Verification items for the finished model (mm, model axes). Face numbers are marked on the shaded views. Give positions to 0.01 mm unless a question says otherwise; leave off trailing zeros. Order: outer loops, then holes, each group sorted by start corner. A loop starts at its lowest first (then second) coordinate and runs counter-clockwise, first axis right, second up.
from build123d import *

# Parameters (mm, degrees)
F1_DEPTH = 100
F2_R     = 15
F3_DEPTH = 100.001
F4_R     = 15
F5_DEPTH = 100.001
F6_R     = 15
F7_DEPTH = 100.001


with BuildPart() as f1:
    # F0 (on Front) → F1 (new body)
    with BuildSketch(Plane.XZ):
        with BuildLine():
            ThreePointArc((46.564883, 30), (40.707019, 44.142136), (26.564883, 50))
            Line((26.564883, 50), (-33.435117, 50))
            ThreePointArc((-33.435117, 50), (-47.577252, 44.142136), (-53.435117, 30))
            Line((-53.435117, 30), (-53.435117, -30))
            ThreePointArc((-53.435117, -30), (-47.577252, -44.142136), (-33.435117, -50))
            Line((-33.435117, -50), (26.564883, -50))
            ThreePointArc((26.564883, -50), (40.707019, -44.142136), (46.564883, -30))
            Line((46.564883, -30), (46.564883, 30))
        make_face()
    extrude(amount=F1_DEPTH)

    # F2 (on face) → F3 (cut, through all)
    with BuildSketch(Plane.XY.offset(50)):
        with Locations((0, -50)):
            Circle(F2_R)
    extrude(amount=-F3_DEPTH, mode=Mode.SUBTRACT)

    # F4 (on face) → F5 (cut, through all)
    with BuildSketch(Plane(origin=(0, 0, 0), x_dir=(-1, 0, 0), z_dir=(0, 1, 0))):
        Circle(F4_R)
    extrude(amount=-F5_DEPTH, mode=Mode.SUBTRACT)

    # F6 (on face) → F7 (cut, through all)
    with BuildSketch(Plane.YZ.offset(46.564883)):
        with Locations((-50, 0)):
            Circle(F6_R)
    extrude(amount=-F7_DEPTH, mode=Mode.SUBTRACT)


solid = f1.part
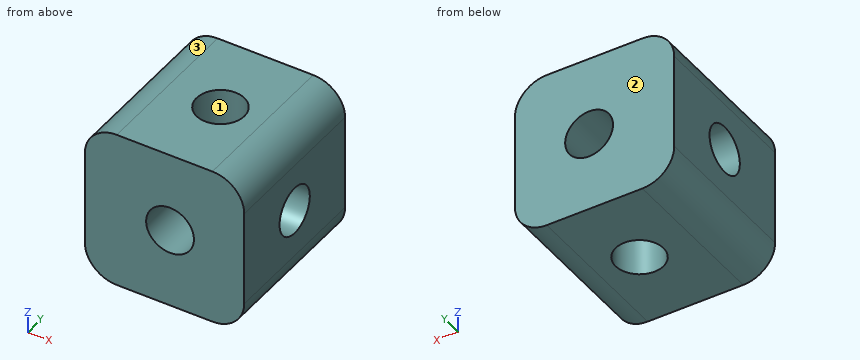
(1) Release check for a two-part mould opening along Y. For the marked faces 1, 2 and 3 record: pulls with the +Y half, pulls with the -Y half, needs draft (parallel to the pull), parting line crosses it, or undercut.
Solved:
face 1: undercut
face 2: pulls with the +Y half
face 3: needs draft
(2) Scan lines: line 1 (Z direction, x = 0, y = -85.5); line 2 (X direction, y = -15, z = 0); line 3 (Y direction, x = 0, z = 29). Record each from-to range of solid material in increasing order.
Solved:
line 1: z = -50 to -15, 15 to 50
line 2: x = -53.44 to -15, 15 to 46.56
line 3: y = -100 to -65, -35 to 0
(3) Section check A-A, the plane y = -50. Enter the section's corners in (x, z), then the cut area to 3 significant figures.
Solved:
outline: (-53.44, -30) arc R20 ccw to (-33.44, -50) - (-15, -50) - (-15, -15) - (-53.44, -15) - close; (-53.44, 15) - (-15, 15) - (-15, 50) - (-33.44, 50) arc R20 ccw to (-53.44, 30) - close; (15, -50) - (26.56, -50) arc R20 ccw to (46.56, -30) - (46.56, -15) - (15, -15) - close; (15, 15) - (46.56, 15) - (46.56, 30) arc R20 ccw to (26.56, 50) - (15, 50) - close
area: 4,560 mm2
(4) Section check D-D, the plane y = -14. Enter the section's corners in (x, z).
Solved:
outline: (-53.44, -30) arc R20 ccw to (-33.44, -50) - (26.56, -50) arc R20 ccw to (46.56, -30) - (46.56, 30) arc R20 ccw to (26.56, 50) - (-33.44, 50) arc R20 ccw to (-53.44, 30) - close; hole circle Ø30 at (0, 0)
(5) Section check C-C, the plane z = 0. Enter the section's corners in (x, y).
Solved:
outline: (-53.44, -100) - (-15, -100) - (-15, -65) - (-53.44, -65) - close; (-53.44, -35) - (-15, -35) - (-15, 0) - (-53.44, 0) - close; (15, -100) - (46.56, -100) - (46.56, -65) - (15, -65) - close; (15, -35) - (46.56, -35) - (46.56, 0) - (15, 0) - close
(6) Go/stop test with flat-tipped pins: pin 1 (1 mm diameter, centred on y = -33, z = 33.5, fed in from -X); pin 2 (24 mm diameter, centred on y = -50, z = 0, fed in from -X) (1 decimal). Record where each tip stops, or that it passes through.
Solved:
pin 1: stops at x = -53.21
pin 2: passes through
(7) Section check B-B, the plane x = -25.5. Enter the section's corners in (y, z).
Solved:
outline: (-100, -50) - (0, -50) - (0, 50) - (-100, 50) - close; hole circle Ø30 at (-50, 0)
